from build123d import *

# Parameters (mm, degrees)
BOSS_EXTRUDE1_DEPTH = 5
SKETCH3_W           = 120
SKETCH3_H           = 6
BOSS_EXTRUDE2_DEPTH = 10
SKETCH5_W           = 24
SKETCH5_H           = 6
CUT_EXTRUDE1_DEPTH  = 10
CUT_EXTRUDE2_START  = -5
SKETCH7_R           = 2.5
CUT_EXTRUDE2_DEPTH  = 25
SKETCH8_R           = 1.25
CUT_EXTRUDE3_DEPTH  = 20
SKETCH9_R           = 1.25
CUT_EXTRUDE4_DEPTH  = 10


with BuildPart() as part:
    # Sketch1 → Boss-Extrude1 (new, symmetric)
    with BuildSketch(Plane(origin=(0, 0, 0), x_dir=(1, 0, 0), z_dir=(0, 1, 0))):
        Polygon((58.46437743, 9.875), (57.15507132, 9.875), (55.92667178, 13.25), (54.980387995, 13.25), (53.751988455, 9.875), (52.442682345, 9.875), (51.214282805, 13.25), (50.26799902, 13.25), (49.03959948, 9.875), (47.73029337, 9.875), (46.50189383, 13.25), (45.555610045, 13.25), (44.327210505, 9.875), (43.017904395, 9.875), (41.789504855, 13.25), (40.84322107, 13.25), (39.61482153, 9.875), (38.30551542, 9.875), (37.07711588, 13.25), (36.130832095, 13.25), (34.902432555, 9.875), (33.593126445, 9.875), (32.364726905, 13.25), (31.41844312, 13.25), (30.19004358, 9.875), (28.88073747, 9.875), (27.65233793, 13.25), (26.706054145, 13.25), (25.477654605, 9.875), (24.168348495, 9.875), (22.939948955, 13.25), (21.99366517, 13.25), (20.76526563, 9.875), (19.45595952, 9.875), (18.22755998, 13.25), (17.281276195, 13.25), (16.052876655, 9.875), (14.743570545, 9.875), (13.515171005, 13.25), (12.56888722, 13.25), (11.34048768, 9.875), (10.03118157, 9.875), (8.80278203, 13.25), (7.856498245, 13.25), (6.628098705, 9.875), (5.318792595, 9.875), (4.090393055, 13.25), (3.14410927, 13.25), (1.91570973, 9.875), (0.60640362, 9.875), (-0.62199592, 13.25), (-1.568279705, 13.25), (-2.796679245, 9.875), (-4.105985355, 9.875), (-5.334384895, 13.25), (-6.28066868, 13.25), (-7.50906822, 9.875), (-8.81837433, 9.875), (-10.04677387, 13.25), (-10.993057655, 13.25), (-12.221457195, 9.875), (-13.530763305, 9.875), (-14.759162845, 13.25), (-15.70544663, 13.25), (-16.93384617, 9.875), (-18.24315228, 9.875), (-19.47155182, 13.25), (-20.417835605, 13.25), (-21.646235145, 9.875), (-22.955541255, 9.875), (-24.183940795, 13.25), (-25.13022458, 13.25), (-26.35862412, 9.875), (-27.66793023, 9.875), (-28.89632977, 13.25), (-29.842613555, 13.25), (-31.071013095, 9.875), (-32.380319205, 9.875), (-33.608718745, 13.25), (-34.55500253, 13.25), (-35.78340207, 9.875), (-37.09270818, 9.875), (-38.32110772, 13.25), (-39.267391505, 13.25), (-40.495791045, 9.875), (-41.805097155, 9.875), (-43.033496695, 13.25), (-43.97978048, 13.25), (-45.20818002, 9.875), (-46.51748613, 9.875), (-47.74588567, 13.25), (-48.692169455, 13.25), (-49.920568995, 9.875), (-51.229875105, 9.875), (-52.458274645, 13.25), (-53.40455843, 13.25), (-54.63295797, 9.875), (-55.94226408, 9.875), (-57.17066362, 13.25), (-58.116947405, 13.25), (-59.345346945, 9.875), (-60, 9.875), (-60, -13.25), (60, -13.25), (60, 13.25), (59.69277697, 13.25), align=None)
    extrude(amount=BOSS_EXTRUDE1_DEPTH, both=True)

    # Sketch3 → Boss-Extrude2 (add)
    with BuildSketch(Plane(origin=(0, 5, 0), x_dir=(1, 0, 0), z_dir=(0, 1, 0))):
        with Locations((0, -16.25)):
            Rectangle(SKETCH3_W, SKETCH3_H)
    extrude(amount=-BOSS_EXTRUDE2_DEPTH)

    # Sketch5 → Cut-Extrude1 (cut)
    with BuildSketch(Plane(origin=(0, 5, 0), x_dir=(1, 0, 0), z_dir=(0, 1, 0))):
        with Locations((-40, -9.932851702)):
            Rectangle(SKETCH5_W, SKETCH5_H)
        with Locations((40, -9.932851702)):
            Rectangle(SKETCH5_W, SKETCH5_H)
    extrude(amount=-CUT_EXTRUDE1_DEPTH, mode=Mode.SUBTRACT)

    # Sketch7 → Cut-Extrude2 (cut)
    with BuildSketch(Plane.XY.offset(6.932851702).offset(CUT_EXTRUDE2_START)):
        with Locations((-40.495791045, 0)):
            Circle(SKETCH7_R)
    cut_extrude2 = extrude(amount=CUT_EXTRUDE2_DEPTH, mode=Mode.SUBTRACT)

    # Mirror1: Cut-Extrude2 across plane
    add(cut_extrude2.mirror(Plane(origin=(0, 0, 0), x_dir=(0, 0, 1), z_dir=(1, 0, 0))), mode=Mode.SUBTRACT)

    # Sketch8 → Cut-Extrude3 (cut)
    with BuildSketch(Plane(origin=(0, 5, 0), x_dir=(1, 0, 0), z_dir=(0, 1, 0))):
        with Locations(Location((-54.081860638, 0.75, 0), (0, 0, 270))):
            Circle(SKETCH8_R)
        with Locations(Location((-45.918139363, 0.75, 0), (0, 0, 270))):
            Circle(SKETCH8_R)
    extrude(amount=-CUT_EXTRUDE3_DEPTH, mode=Mode.SUBTRACT)

    # Sketch9 → Cut-Extrude4 (cut)
    with BuildSketch(Plane(origin=(0, 5, 0), x_dir=(1, 0, 0), z_dir=(0, 1, 0))):
        with Locations(Location((-50, 5.147546331, 0), (0, 0, 270))):
            Circle(SKETCH9_R)
    extrude(amount=-CUT_EXTRUDE4_DEPTH, mode=Mode.SUBTRACT)


solid = part.part
The listing builds one solid part. Answer for the finished solid, in the listing's coordinates (mm). A direction names the side the tool comes from. Coordinates: 2 decimals unless noted, no trailing zeros. Write each loop counter-clockwise with the first axis right and the second up, starting at its lowest first coordinate (ties: lowest second). Pieces come first, ordered by that corner, then holes. Notation, with made-up numbers: (69.25, 41) - (84.25, 41) arc R22 ccw to (84.25, 78) - close; hole circle Ø3 at (56, 60). An arc over 180 degrees is marked (long way). Answer as CSV lines item,"result".
1. Find section C-C (y = -1.5). Give the number of separate pieces and of enclosed holes in the cut face, plus the area to 3 significant figures.
Computed values:
separate pieces,"1"
enclosed holes,"3"
area,"3,290 mm²"
2. Given P1, Ø0.7, axis at x = 34.5, y = -1, coming from the -Z side (3 decimals); P2, Ø1.5, axis at x = 40.5, y = -1, coming from the +Z side; P3, Ø2, axis at x = -50, z = -5.15, coming from the -Y side; P4, Ø5, axis at x = 45, y = 1, coming from the -Z side, each flat-ended and moving along its own axis, determine where each tip first touches the part or whether it passes through.
Computed values:
P1,"stops at z = -9.875"
P2,"stops at z = 1.93"
P3,"passes through"
P4,"stops at z = -13.25"
3. Find section A-A (z = -0.75). Give the vertices of the cut face in (x, y), plus the area to 3 significant figures.
Computed values:
outline,"(-60, -5) - (-55.33, -5) - (-55.33, 5) - (-60, 5) - close; (-52.83, -5) - (-47.17, -5) - (-47.17, 5) - (-52.83, 5) - close; (-44.67, -5) - (60, -5) - (60, 5) - (-44.67, 5) - close"
area,"1,150 mm²"
4. Determine the mould class of faces 3 (the flat face through (-49.298, 0.07, -11.586)), 4 (the flat face through (60, 0, 3)), 5 (the flat face through (37, 0, 12.933)) for opening direction Z: +Z half, -Z half, draft (parallel to the pull), parting line (faces both ways), or undercut.
Computed values:
face 3,"-Z half"
face 4,"draft"
face 5,"undercut"
5. Find section B-B (z = 10). Give the vertices of the cut face in (x, y).
Computed values:
outline,"(-60, -5) - (-52, -5) - (-52, 5) - (-60, 5) - close; (-28, -5) - (28, -5) - (28, 5) - (-28, 5) - close; (52, -5) - (60, -5) - (60, 5) - (52, 5) - close"
6. A tool of negligible diameter and unlimited length cuts with its end or side. For faces 1 (the flat face through (-28, 0, 10)), 2 (the flat face through (-18.85, 0.07, -11.54)), from which of +Z, -Z, +X, -X, +Y, -Y can it reach the whole face along a straight path? Write none if from no direction.
Computed values:
face 1,"+Y, -Y"
face 2,"-Z, +Y, -Y"
7. Straight lines are drawn through the part: line 1 (X direction, y = 3.25, z = -0.75); line 2 (Z direction, x = -8, y = -2.25) (3 decimals). For each, find the intervals that lie inside material, in ascending order. Write a range as [from, to].
Computed values:
line 1,"x = [-60, -55.33], [-52.83, -47.17], [-44.67, 60]"
line 2,"z = [-9.875, 19.25]"
